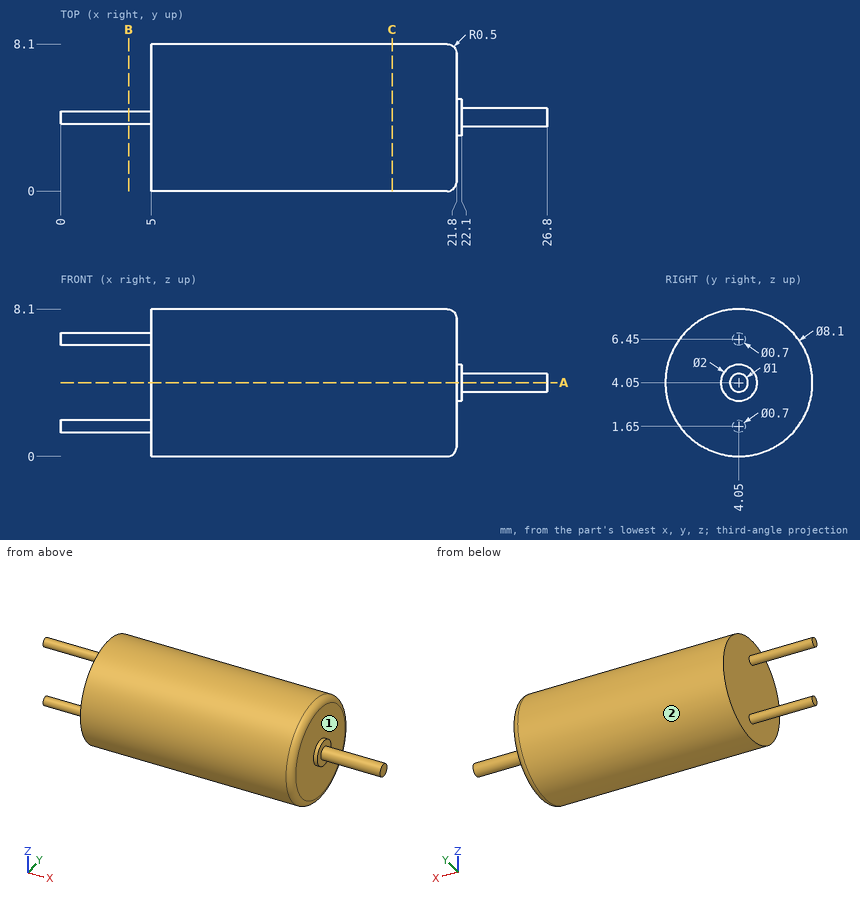
Here's the drawing with two shaded views (mm, measured from the low corner). I have some questions. Give positions to 0.01 mm unless a question says otherwise; leave off trailing zeros. Loops run counter-clockwise (first coordinate to the right, second up) from the corner with the lowest first, then second, coordinate; pieces in that order, holes last. Notation, with made-up numbers: (57.25, -32.75) - (67.25, -32.75) arc R12 cw to (67.25, -15.75) - close; hole circle Ø8 at (68, 15). An arc over 180 degrees is marked (long way). One line per item, written item: value.
(1) If we mould it in two halves opening along Y, with no side actions, what happens to the marked faces 1 and 2? For each: released by +Y, released by -Y, zero draft, split by the parting line, or undercut.
Verdict:
face 1: zero draft
face 2: split by the parting line
(2) If we section it at C-C, the plane x = 18.25: List the corners of the cut face in (y, z) for me.
Verdict:
outline: circle Ø8.1 at (4.05, 4.05)
(3) I'm going to push flat-ended pins straight in: pin 1 (4 mm diameter, centred on y = 1.5, z = 5, fed in from +X); pin 2 (3 mm diameter, centred on x = 7.5, y = 7, fed in from +Z); pin 3 (1.5 mm diameter, centred on y = 3, z = 5, fed in from -X). Where does each tip first touch, or does it pass through?
Verdict:
pin 1: x = 22.1
pin 2: z = 7.83
pin 3: x = 5
(4) If we section it at B-B, the plane x = 3.75: List the corners of the cut face in (y, z) for me.
Verdict:
outline: circle Ø0.7 at (4.05, 1.65); circle Ø0.7 at (4.05, 6.45)
(5) I need wall thicknesses on line 1 along X through (y, z) = (3, 1.5); line 2 along Y through (x, z) = (22.5, 4); line 3 along X through (y, z) = (4.25, 4.25). Which ranges of each line are inside material? Lowest first, please.
Verdict:
line 1: 5 to 21.8
line 2: 3.55 to 4.55
line 3: 5 to 26.8
(6) If we section it at A-A, the plane z = 4.05: List the corners of the cut face in (x, y) for me.
Verdict:
outline: (5, 0) - (21.3, 0) arc R0.5 ccw to (21.8, 0.5) - (21.8, 3.05) - (22.1, 3.05) - (22.1, 3.55) - (26.8, 3.55) - (26.8, 4.55) - (22.1, 4.55) - (22.1, 5.05) - (21.8, 5.05) - (21.8, 7.6) arc R0.5 ccw to (21.3, 8.1) - (5, 8.1) - close
